Here's how the part is built. I have some questions about the finished solid (model axes, mm). A direction names the side the tool comes from. Coordinates: 2 decimals unless noted, no trailing zeros. Write each loop counter-clockwise with the first axis right and the second up, starting at its lowest first coordinate (ties: lowest second). Pieces come first, ordered by that corner, then holes. Notation, with made-up numbers: (32.5, -38.5) -> (85.5, -38.5) arc R31 ccw to (85.5, 0.5) -> close; hole circle Ø6 at (-26, 40). An arc over 180 degrees is marked (long way). Put each result on its own line as item: value.
```python
from build123d import *

# Parameters (mm, degrees)
SKETCH1_W               = 7
SKETCH1_H               = 7.5
SKETCH2_R               = 2.5
CUT_EXTRUDE1_DEPTH      = 1
CUT_EXTRUDE1_DEPTH_BACK = 17


with BuildPart() as part:
    # Sketch1 → Revolve1 (revolve)
    with BuildSketch(Plane.XY):
        Polygon((-7, 7.5), (-7, 0), (-16, 0), (-16, 7.5), (-15, 7.5), (-15, 5.87), (-8, 5.87), (-8, 7.5), align=None)
        with Locations((-3.5, 3.75)):
            Rectangle(SKETCH1_W, SKETCH1_H)
    revolve(axis=Axis((-7, 0, 0), (-1, 0, 0)))

    # Sketch2 → Cut-Extrude1 (cut, two sides)
    with BuildSketch(Plane.ZY.offset(16)) as cut_extrude1_sk:
        Circle(SKETCH2_R)
    extrude(amount=CUT_EXTRUDE1_DEPTH, mode=Mode.SUBTRACT)
    extrude(cut_extrude1_sk.sketch, amount=-CUT_EXTRUDE1_DEPTH_BACK, mode=Mode.SUBTRACT)


solid = part.part
```
Item 1: Please list where these lines run through material, in increasing order: line 1 along X through (y, z) = (-6.25, -1); line 2 along Y through (x, z) = (-6, 0); line 3 along Y through (x, z) = (-10.5, 0). Write a range as from..to.
Output:
line 1: x = -16..-15, -8..0
line 2: y = -7.5..-2.5, 2.5..7.5
line 3: y = -5.87..-2.5, 2.5..5.87
Item 2: For P1, Ø1.5, axis at x = -6, y = -1.5, coming from the +Z side, with a flat end and sliding along its axis, tell me the tip position at first contact or that it passes through.
Output:
P1: stops at z = 7.46
Item 3: Imagine slicing it at D-D on y = 5. Write out the boundary of the cut face in (x, z), then the cut area to 3 significant figures.
Output:
outline: (-16, -5.59) -> (-15, -5.59) -> (-15, -3.08) -> (-8, -3.08) -> (-8, -5.59) -> (0, -5.59) -> (0, 5.59) -> (-8, 5.59) -> (-8, 3.08) -> (-15, 3.08) -> (-15, 5.59) -> (-16, 5.59) -> close
area: 144 mm²
Item 4: If we mould it in two halves opening along X, with no side actions, what happens to faces 1 (the flat face through (0, 2, -2)), 2 (the cylindrical face through (-8.11, -2.44, -0.54)), 3 (the flat face through (-15, -5.04, 3.3))? For each: released by +X, released by -X, zero draft, split by the parting line, or undercut.
Output:
face 1: released by +X
face 2: zero draft
face 3: undercut
Item 5: Which directions (+Z, -Z, +X, -X, +Y, -Y) give clear straight access to the entire face, cutting with the end or side of a thin tool? Please do faces 4 (the cylindrical face through (-4.056, -7.493, -0.33)), 5 (the cylindrical face through (-11.451, -4.326, -3.967)).
Output:
face 4: +X, -X
face 5: none
Item 6: Imagine slicing it at A-A on z = 0. Write out the boundary of the cut face in (x, y), then the cut area to 3 significant figures.
Output:
outline: (-16, -7.5) -> (-15, -7.5) -> (-15, -5.87) -> (-8, -5.87) -> (-8, -7.5) -> (0, -7.5) -> (0, -2.5) -> (-16, -2.5) -> close; (-16, 2.5) -> (0, 2.5) -> (0, 7.5) -> (-8, 7.5) -> (-8, 5.87) -> (-15, 5.87) -> (-15, 7.5) -> (-16, 7.5) -> close
area: 137 mm²
Item 7: Imagine slicing it at C-C on x = -11.5. Write out the boundary of the cut face in (y, z).
Output:
outline: circle Ø11.74 at (0, 0); hole circle Ø5 at (0, 0)
